```python
from build123d import *

# Parameters (mm, degrees)
F1_DEPTH  = 76.2
F2_T      = -3.175
F4_DEPTH  = 25.4
F5_W      = 127
F5_H      = 25.4
F6_DEPTH  = 25.4
F7_W      = 330.2
F7_H      = 127
F8_DEPTH  = 3.175
F9_W      = 101.6
F9_H      = 127
F10_DEPTH = 25.4


# Not quite as in the source:
# - a pattern or mirror of a feature is missing from the dataset's text; its kind, count and spacing are read off the source's solid


with BuildPart() as f1:
    # F0 (on Front) → F1 (new body)
    with BuildSketch(Plane.XZ):
        with BuildLine():
            ThreePointArc((-1.539e-07, -127), (89.8025611563, -89.8025612651), (127, 0))
            ThreePointArc((127, 0), (89.8025612186, 89.8025612028), (2.24e-08, 127))
            ThreePointArc((2.24e-08, 127), (-127, 8.82e-08), (-1.539e-07, -127))
        make_face()
        with BuildLine():
            ThreePointArc((2.24e-08, 127), (89.8025612186, 89.8025612028), (127, 0))
            ThreePointArc((127, 0), (89.8025611563, -89.8025612651), (-1.539e-07, -127))
            Line((-1.539e-07, -127), (165.1, -127))
            Line((165.1, -127), (165.1, 127))
            Line((165.1, 127), (2.24e-08, 127))
        make_face()
        with BuildLine():
            ThreePointArc((-1.539e-07, -127), (-127, 8.82e-08), (2.24e-08, 127))
            Line((2.24e-08, 127), (-165.1, 127))
            Line((-165.1, 127), (-165.1, -127))
            Line((-165.1, -127), (-1.539e-07, -127))
        make_face()
        Polygon((165.1, -127), (-1.539e-07, -127), (-165.1, -127), (-76.2, -189.2484501468), (76.2, -189.2484501468), align=None)
    extrude(amount=F1_DEPTH)

    # F2
    f2_openings = [f1.faces().sort_by_distance(p)[0] for p in [
        (0, -38.1, 127),
    ]]
    offset(amount=F2_T, openings=f2_openings)

    # F3 (on face) → F4 (cut)
    with BuildSketch(Plane.XZ.offset(76.2)):
        Polygon((0, -76.2), (0, 127), (-50.8, 127), (-50.8, -50.8), align=None)
    f4 = extrude(amount=-F4_DEPTH, mode=Mode.SUBTRACT)

    # F4_copies: F4 across plane
    add(f4.mirror(Plane(origin=(0, 0, 0), x_dir=(0, 0, 1), z_dir=(1, 0, 0))), mode=Mode.SUBTRACT)

    # F5 (on face) → F6 (cut)
    with BuildSketch(Plane.XZ.offset(3.175)):
        with Locations((0, 127)):
            Rectangle(F5_W, F5_H)
    extrude(amount=-F6_DEPTH, mode=Mode.SUBTRACT)

    # F7 (on face) → F8 (join)
    with BuildSketch(Plane.XZ.offset(76.2)):
        with Locations((0, 190.5)):
            Rectangle(F7_W, F7_H)
    extrude(amount=-F8_DEPTH)

    # F9 (on face) → F10 (cut)
    with BuildSketch(Plane.XZ.offset(76.2)):
        with Locations((0, 190.5)):
            Rectangle(F9_W, F9_H)
    extrude(amount=-F10_DEPTH, mode=Mode.SUBTRACT)


solid = f1.part
```
The listing builds one solid part. Answer for the finished solid, in the listing's coordinates (mm). A direction names the side the tool comes from. Give positions to 0.01 mm unless a question says otherwise; leave off trailing zeros. Write each loop counter-clockwise with the first axis right and the second up, starting at its lowest first coordinate (ties: lowest second). Pieces come first, ordered by that corner, then holes. Notation, with made-up numbers: (-3.75, 70) - (35.25, 70) arc R15 ccw to (35.25, 85) - close; hole circle Ø7 at (53.25, 4.5). An arc over 180 degrees is marked (long way). Use one line per item in the form item = value. Start each with the question number.
1) Consider line 1 along Y through (x, z) = (119.5, -26.5) (3 decimals); line 2 along X through (y, z) = (-51.5, -118.5) (3 decimals); line 3 along Y through (x, z) = (139, 200) (3 decimals). Determine where each line is inside the solid, lowest interval first. Write a range as from..to.
2) Find section B-B on z = 210. Determine the outline of the cut face in (x, y) (3 decimals), plus the area to 3 significant figures.
3) Find section D-D on x = 14.5. Determine the outline of the cut face in (y, z) (3 decimals), plus the area to 3 significant figures.
4) Flat-ended cylindrical pins translate along their axes: pin 1 Ø21 at (x, y) = (1, -43.5) entering from +Z; pin 2 Ø8 at (x, y) = (-114, -28) entering from +Z; pin 3 Ø2.5 at (x, y) = (4.5, -1) entering from +Z. Find the tip coordinate at first contact, or state that the pin passes through.
5) Find section A-A on z = -105.5. Determine the outline of the cut face in (x, y) (3 decimals), plus the area to 3 significant figures.
6) Find section C-C on y = -39.5. Determine the outline of the cut face in (x, z) (3 decimals), plus the area to 3 significant figures.
7) A tool of negligible diameter and unlimited length cuts with its end or side. For faces 4 (the face through (137, -1, 127)), 5 (the face through (-2, 0, -29)), 6 (the face through (-165.1, -39, 18)), 7 (the face through (-76, -73.025, 37)), 8 (the face through (25.8, -74.6, -63.3)), from which of +Z, -Z, +X, -X, +Y, -Y can it reach the whole face along a straight path? Write none if from no direction.
8) The mould has two halves that part along Y. Classify faces 1 (the face through (-76, -76.2, 35)), 2 (the face through (-2, -3.175, -27)), 3 (the face through (-121.27, -37.57, -157.69)): pulls with the +Y half, pulls with the -Y half, needs draft (parallel to the pull), parting line crosses it, or undercut.
Geometry results:
q1.line_1 = -76.2..-73.025, -3.175..0
q1.line_2 = -165.1..-161.925, 161.925..165.1
q1.line_3 = -76.2..-73.025
q2.outline = (-165.1, -76.2) - (-50.8, -76.2) - (-50.8, -73.025) - (-165.1, -73.025) - close; (50.8, -76.2) - (165.1, -76.2) - (165.1, -73.025) - (50.8, -73.025) - close
q2.area = 726 mm2
q3.outline = (-76.2, -189.248) - (0, -189.248) - (0, 114.3) - (-3.175, 114.3) - (-3.175, -186.073) - (-73.025, -186.073) - (-73.025, -68.95) - (-76.2, -68.95) - close
q3.area = 1,570 mm2
q4.pin_1 = -186.07
q4.pin_2 = -156.1
q4.pin_3 = 114.3
q5.outline = (-165.1, -76.2) - (165.1, -76.2) - (165.1, 0) - (-165.1, 0) - close; hole (-161.925, -73.025) - (161.925, -73.025) - (161.925, -3.175) - (-161.925, -3.175) - close
q5.area = 2,540 mm2
q6.outline = (-165.1, -127) - (-76.2, -189.248) - (76.2, -189.248) - (165.1, -127) - (165.1, 127) - (161.925, 127) - (161.925, -125.347) - (75.199, -186.073) - (-75.199, -186.073) - (-161.925, -125.347) - (-161.925, 127) - (-165.1, 127) - close
q6.area = 2,770 mm2
q7.face_4 = +Z, +X, -X, +Y
q7.face_5 = +Z, -Z, +X, -X, +Y
q7.face_6 = +Z, -Z, -X, +Y, -Y
q7.face_7 = +Z
q7.face_8 = +Z, -Y
q8.face_1 = pulls with the -Y half
q8.face_2 = undercut
q8.face_3 = needs draft
